from build123d import *

# Parameters (mm, degrees)
SKETCH1_W                      = 20.045
SKETCH1_H                      = 20.045
BOSS_EXTRUDE1_DEPTH            = 73.5
CUT_EXTRUDE2_DEPTH             = 108.652129543
SKETCH3_RX                     = 9
SKETCH3_RY                     = 5
CUT_EXTRUDE4_DEPTH             = 108.652129543
CUT_EXTRUDE5_DEPTH             = 108.652129714
CUT_EXTRUDE5_DEPTH_BACK        = 108.652129714
SKETCH4_R                      = 7
SKETCH5_R                      = 7
CUT_EXTRUDE6_DEPTH             = 10
CUT_EXTRUDE7_START             = -10
SKETCH6_R                      = 7
CUT_EXTRUDE7_DEPTH             = 10
SKETCH7_R                      = 7.5
CUT_EXTRUDE8_DEPTH             = 10
SKETCH8_R                      = 7
CUT_EXTRUDE9_DEPTH             = 108.652129714
CUT_EXTRUDE9_DIRECTION_2_REACH = 109.652
SKETCH9_R                      = 2.75
CUT_EXTRUDE10_DEPTH            = 15
SKETCH10_R                     = 5.1
CUT_EXTRUDE11_DEPTH            = 4
SKETCH11_W                     = 20.045
SKETCH11_H                     = 20.045
BOSS_EXTRUDE2_DEPTH            = 73.5


with BuildPart() as part:
    # Sketch1 → Boss-Extrude1 (new body)
    with BuildSketch(Plane.XY):
        Polygon((59.861803254, -23.0225), (50.316348709, -51.0225), (-50.316348709, -51.0225), (-59.861803254, -23.0225), (-38.0225, -18.146810718), (-38.0225, 11.146810718), (-10.0225, 20.692265263), (0, 20.692265263), (10.0225, 20.692265263), (38.0225, 11.146810718), (38.0225, -18.146810718), align=None)
        Rectangle(SKETCH1_W, SKETCH1_H, mode=Mode.SUBTRACT)
        Polygon((-12.5, -26.0225), (12.5, -26.0225), (20, -48.0225), (-20, -48.0225), align=None, mode=Mode.SUBTRACT)
        Polygon((15.669537991, -26.0225), (23.169537991, -48.0225), (48.169537991, -48.0225), (55.669537991, -26.0225), align=None, mode=Mode.SUBTRACT)
        Polygon((-15.669537991, -26.0225), (-55.669537991, -26.0225), (-48.169537991, -48.0225), (-23.169537991, -48.0225), align=None, mode=Mode.SUBTRACT)
        Polygon((-13.0225, -23.5), (-13.0225, 16.5), (-35.0225, 9), (-35.0225, -16), align=None, mode=Mode.SUBTRACT)
        Polygon((35.0225, 9), (35.0225, -16), (13.0225, -23.5), (13.0225, 16.5), align=None, mode=Mode.SUBTRACT)
    extrude(amount=BOSS_EXTRUDE1_DEPTH)

    # Sketch2 → Cut-Extrude2 (cut, through all)
    with BuildSketch(Plane.XY):
        Polygon((-17.68804096, -24.0225), (-55.162041129, -24.0225), (-32.517435529, -18.967024579), align=None)
        Polygon((17.68804096, -24.0225), (55.162041129, -24.0225), (32.517435529, -18.967024579), align=None)
    extrude(amount=CUT_EXTRUDE2_DEPTH, mode=Mode.SUBTRACT)

    # Sketch3 → Cut-Extrude4 (cut, through all)
    with BuildSketch(Plane.XY):
        with Locations((0, -18)):
            Ellipse(SKETCH3_RX, SKETCH3_RY)
    extrude(amount=CUT_EXTRUDE4_DEPTH, mode=Mode.SUBTRACT)

    # Sketch4 → Cut-Extrude5 (cut, two sides: drawn at the far end of the back side and taken through both)
    with BuildSketch(Plane(origin=(0, 0, 0), x_dir=(0, 0, -1), z_dir=(1, 0, 0)).offset(-CUT_EXTRUDE5_DEPTH_BACK)):
        with Locations(Location((-36.75, -36.52, 0), (0, 0, 270))):
            Circle(SKETCH4_R)
        with Locations(Location((-58.75, -36.52, 0), (0, 0, 270))):
            Circle(SKETCH4_R)
        with Locations(Location((-14.75, -36.52, 0), (0, 0, 270))):
            Circle(SKETCH4_R)
    extrude(amount=CUT_EXTRUDE5_DEPTH + CUT_EXTRUDE5_DEPTH_BACK, mode=Mode.SUBTRACT)

    # Sketch5 → Cut-Extrude6 (cut)
    with BuildSketch(Plane(origin=(38.0225, 0, 0), x_dir=(0, 0, -1), z_dir=(1, 0, 0))):
        with Locations(Location((-36.75, -3.5, 0), (0, 0, 90))):
            Circle(SKETCH5_R)
        with Locations(Location((-14.75, -3.5, 0), (0, 0, 90))):
            Circle(SKETCH5_R)
        with Locations(Location((-58.75, -3.5, 0), (0, 0, 90))):
            Circle(SKETCH5_R)
    extrude(amount=-CUT_EXTRUDE6_DEPTH, mode=Mode.SUBTRACT)

    # Sketch6 → Cut-Extrude7 (cut)
    with BuildSketch(Plane.ZY.offset(38.0225).offset(CUT_EXTRUDE7_START)):
        with Locations(Location((36.75, -3.5, 0), (0, 0, 90))):
            Circle(SKETCH6_R)
        with Locations(Location((58.75, -3.5, 0), (0, 0, 90))):
            Circle(SKETCH6_R)
        with Locations(Location((14.75, -3.5, 0), (0, 0, 90))):
            Circle(SKETCH6_R)
    extrude(amount=CUT_EXTRUDE7_DEPTH, mode=Mode.SUBTRACT)

    # Sketch7 → Cut-Extrude8 (cut)
    with BuildSketch(Plane.XZ.offset(51.0225)):
        with Locations((0, 36.75)):
            Circle(SKETCH7_R)
        with Locations((35.16, 36.75)):
            Circle(SKETCH7_R)
        with Locations((-35.16, 36.75)):
            Circle(SKETCH7_R)
        with Locations((0, 58.75)):
            Circle(SKETCH7_R)
        with Locations((35.16, 58.75)):
            Circle(SKETCH7_R)
        with Locations((-35.16, 58.75)):
            Circle(SKETCH7_R)
        with Locations((0, 14.75)):
            Circle(SKETCH7_R)
        with Locations((35.16, 14.75)):
            Circle(SKETCH7_R)
        with Locations((-35.16, 14.75)):
            Circle(SKETCH7_R)
    extrude(amount=-CUT_EXTRUDE8_DEPTH, mode=Mode.SUBTRACT)

    # Sketch8 → Cut-Extrude9 (cut)
    with BuildSketch(Plane(origin=(0, 0, 0), x_dir=(1, 0, 0), z_dir=(0, 1, 0))):
        with Locations(Location((23.52, -36.75, 0), (0, 0, 146.422345946))):
            Circle(SKETCH8_R)
        with Locations(Location((23.52, -14.75, 0), (0, 0, 146.422345946))):
            Circle(SKETCH8_R)
        with Locations(Location((23.52, -58.75, 0), (0, 0, 146.422345946))):
            Circle(SKETCH8_R)
        with Locations(Location((-23.52, -58.75, 0), (0, 0, 33.577654054))):
            Circle(SKETCH8_R)
        with Locations(Location((-23.52, -14.75, 0), (0, 0, 33.577654054))):
            Circle(SKETCH8_R)
        with Locations(Location((-23.52, -36.75, 0), (0, 0, 33.577654054))):
            Circle(SKETCH8_R)
    extrude(amount=CUT_EXTRUDE9_DEPTH, mode=Mode.SUBTRACT)

    # Cut-Extrude9 direction 2: up to this face of the body (flat: up to its plane)
    cut_extrude9_direction_2_end = Plane(part.part.faces().sort_by_distance((-36.425041044, -24.0225, 36.75))[0])
    # Sketch8 → Cut-Extrude9 direction 2 (cut, up to the picked face)
    with BuildSketch(Plane(origin=(0, 0, 0), x_dir=(1, 0, 0), z_dir=(0, 1, 0)), mode=Mode.PRIVATE) as cut_extrude9_direction_2_sk1:
        with Locations(Location((23.52, -36.75, 0), (0, 0, 146.422345946))):
            Circle(SKETCH8_R)
    cut_extrude9_direction_2_tool1 = split(extrude(cut_extrude9_direction_2_sk1.sketch, amount=-CUT_EXTRUDE9_DIRECTION_2_REACH, mode=Mode.PRIVATE), bisect_by=cut_extrude9_direction_2_end, keep=Keep.BOTH, mode=Mode.PRIVATE)
    # Sketch8 → Cut-Extrude9 direction 2 (cut, up to the picked face)
    with BuildSketch(Plane(origin=(0, 0, 0), x_dir=(1, 0, 0), z_dir=(0, 1, 0)), mode=Mode.PRIVATE) as cut_extrude9_direction_2_sk2:
        with Locations(Location((23.52, -14.75, 0), (0, 0, 146.422345946))):
            Circle(SKETCH8_R)
    cut_extrude9_direction_2_tool2 = split(extrude(cut_extrude9_direction_2_sk2.sketch, amount=-CUT_EXTRUDE9_DIRECTION_2_REACH, mode=Mode.PRIVATE), bisect_by=cut_extrude9_direction_2_end, keep=Keep.BOTH, mode=Mode.PRIVATE)
    # Sketch8 → Cut-Extrude9 direction 2 (cut, up to the picked face)
    with BuildSketch(Plane(origin=(0, 0, 0), x_dir=(1, 0, 0), z_dir=(0, 1, 0)), mode=Mode.PRIVATE) as cut_extrude9_direction_2_sk3:
        with Locations(Location((23.52, -58.75, 0), (0, 0, 146.422345946))):
            Circle(SKETCH8_R)
    cut_extrude9_direction_2_tool3 = split(extrude(cut_extrude9_direction_2_sk3.sketch, amount=-CUT_EXTRUDE9_DIRECTION_2_REACH, mode=Mode.PRIVATE), bisect_by=cut_extrude9_direction_2_end, keep=Keep.BOTH, mode=Mode.PRIVATE)
    # Sketch8 → Cut-Extrude9 direction 2 (cut, up to the picked face)
    with BuildSketch(Plane(origin=(0, 0, 0), x_dir=(1, 0, 0), z_dir=(0, 1, 0)), mode=Mode.PRIVATE) as cut_extrude9_direction_2_sk4:
        with Locations(Location((-23.52, -58.75, 0), (0, 0, 33.577654054))):
            Circle(SKETCH8_R)
    cut_extrude9_direction_2_tool4 = split(extrude(cut_extrude9_direction_2_sk4.sketch, amount=-CUT_EXTRUDE9_DIRECTION_2_REACH, mode=Mode.PRIVATE), bisect_by=cut_extrude9_direction_2_end, keep=Keep.BOTH, mode=Mode.PRIVATE)
    # Sketch8 → Cut-Extrude9 direction 2 (cut, up to the picked face)
    with BuildSketch(Plane(origin=(0, 0, 0), x_dir=(1, 0, 0), z_dir=(0, 1, 0)), mode=Mode.PRIVATE) as cut_extrude9_direction_2_sk5:
        with Locations(Location((-23.52, -14.75, 0), (0, 0, 33.577654054))):
            Circle(SKETCH8_R)
    cut_extrude9_direction_2_tool5 = split(extrude(cut_extrude9_direction_2_sk5.sketch, amount=-CUT_EXTRUDE9_DIRECTION_2_REACH, mode=Mode.PRIVATE), bisect_by=cut_extrude9_direction_2_end, keep=Keep.BOTH, mode=Mode.PRIVATE)
    # Sketch8 → Cut-Extrude9 direction 2 (cut, up to the picked face)
    with BuildSketch(Plane(origin=(0, 0, 0), x_dir=(1, 0, 0), z_dir=(0, 1, 0)), mode=Mode.PRIVATE) as cut_extrude9_direction_2_sk6:
        with Locations(Location((-23.52, -36.75, 0), (0, 0, 33.577654054))):
            Circle(SKETCH8_R)
    cut_extrude9_direction_2_tool6 = split(extrude(cut_extrude9_direction_2_sk6.sketch, amount=-CUT_EXTRUDE9_DIRECTION_2_REACH, mode=Mode.PRIVATE), bisect_by=cut_extrude9_direction_2_end, keep=Keep.BOTH, mode=Mode.PRIVATE)
    add(cut_extrude9_direction_2_tool1.solids().sort_by(Axis((23.52, 0, 36.75), (0, -1, 0)))[0], mode=Mode.SUBTRACT)
    add(cut_extrude9_direction_2_tool2.solids().sort_by(Axis((23.52, 0, 14.75), (0, -1, 0)))[0], mode=Mode.SUBTRACT)
    add(cut_extrude9_direction_2_tool3.solids().sort_by(Axis((23.52, 0, 58.75), (0, -1, 0)))[0], mode=Mode.SUBTRACT)
    add(cut_extrude9_direction_2_tool4.solids().sort_by(Axis((-23.52, 0, 58.75), (0, -1, 0)))[0], mode=Mode.SUBTRACT)
    add(cut_extrude9_direction_2_tool5.solids().sort_by(Axis((-23.52, 0, 14.75), (0, -1, 0)))[0], mode=Mode.SUBTRACT)
    add(cut_extrude9_direction_2_tool6.solids().sort_by(Axis((-23.52, 0, 36.75), (0, -1, 0)))[0], mode=Mode.SUBTRACT)

    # Sketch9 → Cut-Extrude10 (cut)
    with BuildSketch(Plane(origin=(0, 20.692265263, 0), x_dir=(1, 0, 0), z_dir=(0, 1, 0))):
        with Locations(Location((0, -10, 0), (0, 0, 180))):
            Circle(SKETCH9_R)
        with Locations((0, -63.5)):
            Circle(SKETCH9_R)
    extrude(amount=-CUT_EXTRUDE10_DEPTH, mode=Mode.SUBTRACT)

    # Sketch10 → Cut-Extrude11 (cut)
    with BuildSketch(Plane(origin=(0, 20.692265263, 0), x_dir=(1, 0, 0), z_dir=(0, 1, 0))):
        with Locations(Location((0, -10, 0), (0, 0, 180))):
            Circle(SKETCH10_R)
        with Locations(Location((0, -63.5, 0), (0, 0, 180))):
            Circle(SKETCH10_R)
    extrude(amount=-CUT_EXTRUDE11_DEPTH, mode=Mode.SUBTRACT)

    # Sketch11 → Boss-Extrude2 (add)
    with BuildSketch(Plane.XY):
        Polygon((-50.316348709, -51.0225), (-42.816348709, -73.0225), (42.816348709, -73.0225), (50.316348709, -51.0225), (59.861803254, -23.0225), (38.0225, -18.146810718), (38.0225, 11.146810718), (10.0225, 20.692265263), (-10.0225, 20.692265263), (-38.0225, 11.146810718), (-38.0225, -18.146810718), (-59.861803254, -23.0225), align=None)
        Rectangle(SKETCH11_W, SKETCH11_H, mode=Mode.SUBTRACT)
    extrude(amount=BOSS_EXTRUDE2_DEPTH)


solid = part.part
Geometry: final body of the model. Coordinates: model frame, mm. A direction names the side the tool comes from. Coordinates: 2 decimals unless noted, no trailing zeros. Order: outer loops, then holes, each group sorted by start corner. A loop starts at its lowest first (then second) coordinate and runs counter-clockwise, first axis right, second up.
1) Section A-A (z = 59.5). Return loops of the section in (x, y).
Result sheet:
outline: (-59.86, -23.02) - (-42.82, -73.02) - (42.82, -73.02) - (59.86, -23.02) - (38.02, -18.15) - (38.02, 11.15) - (10.02, 20.69) - (-10.02, 20.69) - (-38.02, 11.15) - (-38.02, -18.15) - close; hole (-10.02, -10.02) - (10.02, -10.02) - (10.02, 10.02) - (-10.02, 10.02) - close
2) Ray query, probe 1 along Y at (x, z) = (2.5, 66); probe 2 along X at (y, z) = (-3, 31); probe 3 along X at (y, z) = (-18, 30). Return the intervals inside material, ascending.
Result sheet:
probe 1: y = -73.02 to -10.02, 10.02 to 20.69
probe 2: x = -38.02 to -10.02, 10.02 to 38.02
probe 3: x = -38.02 to 38.02
3) Set-up query: faces 4 (the flat face through (10.022, 0, 36)), 5 (the flat face through (38.022, -3, 36)), 6 (the flat face through (-38.022, -4, 36)). Return all of +Z, -Z, +X, -X, +Y, -Y with unobstructed straight access to the full face (end or side cutting, diameter ignored); none if empty.
Result sheet:
face 4: +Z, -Z
face 5: +Z, -Z, +X, +Y
face 6: +Z, -Z, -X, +Y
4) Section C-C (x = -7). Return loops of the section in (y, z), then the cut area to 3 significant figures.
Result sheet:
outline: (-73.02, 0) - (-10.02, 0) - (-10.02, 73.5) - (-73.02, 73.5) - close; (10.02, 0) - (20.69, 0) - (20.69, 73.5) - (10.02, 73.5) - close
area: 5,410 mm2
5) Section D-D (y = -64). Return loops of the section in (x, z), then the cut area to 3 significant figures.
Result sheet:
outline: (-45.89, 0) - (45.89, 0) - (45.89, 73.5) - (-45.89, 73.5) - close
area: 6,750 mm2
6) Draft query along Y for faces 1 (the flat face through (0, 10.022, 36)), 2 (the flat face through (-1, -36, 0)), 3 (the flat face through (-49.1, -20.62, 36.24)). Return one class per face: released by +Y, released by -Y, zero draft, split by the parting line, or undercut.
Result sheet:
face 1: undercut
face 2: zero draft
face 3: released by +Y
7) Section B-B (y = -2.5). Return loops of the section in (x, z).
Result sheet:
outline: (-38.02, 0) - (-10.02, 0) - (-10.02, 73.5) - (-38.02, 73.5) - close; (10.02, 0) - (38.02, 0) - (38.02, 73.5) - (10.02, 73.5) - close
8) First-contact query: P1, Ø10, axis at y = -4.5, z = 18.5, coming from the -X side; P2, Ø2, axis at x = -34.5, z = 13, coming from the +Y side; P3, Ø14.5, axis at y = 2, z = 49.5, coming from the +X side. Flat tips, straight axial feed; report the tip coordinate or a pass-through.
Result sheet:
P1: stops at x = -38.02
P2: stops at y = 12.69
P3: stops at x = 38.02
